Here's how the part is built. I have some questions about the finished solid (model axes, mm). A direction names the side the tool comes from. Round coordinates to 2 decimals unless told otherwise and drop trailing zeros. Order: outer loops, then holes, each group sorted by start corner. A loop starts at its lowest first (then second) coordinate and runs counter-clockwise, first axis right, second up. Notation, with made-up numbers: (14, 64) -> (30, 64) arc R36 ccw to (30, 98) -> close; hole circle Ø5 at (36, -27). An arc over 180 degrees is marked (long way). Use a Markdown table: item, result. Add a question column.
from build123d import *

# Parameters (mm, degrees)
BOSS_EXTRUDE1_DEPTH = 40
FILLET1_R           = 1
BOSS_EXTRUDE2_DEPTH = 7.5


with BuildPart() as part:
    # Sketch1 → Boss-Extrude1 (new body)
    with BuildSketch(Plane(origin=(0, 0, 0), x_dir=(1, 0, 0), z_dir=(0, 1, 0))):
        Polygon((0, 17.282938314), (-16.6777552, -7.65403186), (13.257172065, -9.628906454), align=None)
        Polygon((-0.263316613, 13.291614679), (-13.089509231, -5.886408918), (9.932242708, -7.405205761), align=None, mode=Mode.SUBTRACT)
    extrude(amount=BOSS_EXTRUDE1_DEPTH)

    # Fillet1
    fillet1_edges = [part.edges().sort_by_distance(p)[0] for p in [
        (9.932242708, 20, 7.405205761),
        (-0.263316613, 20, -13.291614679),
        (-13.089509231, 20, 5.886408918),
        (13.257172065, 20, 9.628906454),
        (-16.6777552, 20, 7.65403186),
        (0, 20, -17.282938314),
    ]]
    fillet(fillet1_edges, radius=FILLET1_R)

    # Sketch2 → Boss-Extrude2 (add, symmetric)
    with BuildSketch(Plane(origin=(0, 20, 0), x_dir=(-1, 0, 0), z_dir=(0, -1, 0))):
        Polygon((18.471878185, -8.537843331), (-14.919636743, -10.740756801), (-0.131658306, 19.278600132), align=None)
        with BuildLine():
            Line((-12.491768879, -8.075150372), (-0.765403186, 15.729182232))
            ThreePointArc((-0.765403186, 15.729182232), (0.065829153, 16.285107406), (0.962890645, 15.84320167))
            Line((0.962890645, 15.84320167), (15.714864555, -6.214295216))
            ThreePointArc((15.714864555, -6.214295216), (15.780693708, -7.212126125), (14.949461369, -7.768051298))
            Line((14.949461369, -7.768051298), (-11.528878233, -9.514887016))
            ThreePointArc((-11.528878233, -9.514887016), (-12.425939725, -9.072981281), (-12.491768879, -8.075150372))
        make_face(mode=Mode.SUBTRACT)
    extrude(amount=BOSS_EXTRUDE2_DEPTH, both=True)


solid = part.part
(1) I'm going to push flat-ended pins straight in: P1, Ø5, axis at y = 22, z = 1, coming from the -X side; P2, Ø10, axis at x = -9.5, y = 4.5, coming from the -Z side; P3, Ø12, axis at y = 23, z = -3.5, coming from the -X side. Where does each tip first touch, or does it pass through?
(2) I want a section at B-B on x = -8. List the corners of the cut face in (y, z) for me.
(3) If we mould it in two halves opening along Z, with no side actions, what happens to faces 5 (the flat face through (-1.9, 6.16, 8.63)), 6 (the cylindrical face through (-15.787, 33.838, 7.199)), 7 (the cylindrical face through (-12.2, 20.28, 5.43)), 8 (the flat face through (7.63, 19.9, -4.06))? For each: pulls with the +Z half, pulls with the -Z half, needs draft (parallel to the pull), parting line crosses it, or undercut.
(4) I want a section at D-D on x = -13. List the corners of the cut face in (y, z) for me, and give its area (3 significant figures).
(5) Please list where these lines run through material, in increasing order: probe 1 along Y at (x, z) = (-16, 7.5); probe 2 along Z at (x, y) = (6, 38.5); probe 3 along Z at (x, y) = (-11.5, 6). Write a range as from..to.
(6) I want a section at C-C on z = -2.5. List the corners of the cut face in (x, y) for me.
(7) I want a section at A-A on y = 12. List the corners of the cut face in (x, z) for me.
(8) On a 3-axis mill with a long thin cutter (end or side, diameter ignored), from which of +Z, -Z, +X, -X, +Y, -Y can I reach the whole of each face in a straight line? I mean faces 1 (the flat face through (6.71, 33.66, -3.66)), 2 (the cylindrical face through (-0.08, 6.338, -16.286)), 3 (the flat face through (-8.236, 33.662, -4.969)), 4 (the flat face through (7, 12.5, -4)). Say none if no direction works.
Output:
| question | item | result |
|---|---|---|
| 1 | P1 | x = -15.1 |
| 1 | P2 | z = -10.55 |
| 1 | P3 | x = -14.43 |
| 2 | outline | (0, -5.32) -> (12.5, -5.32) -> (12.5, -7.12) -> (27.5, -7.12) -> (27.5, -5.32) -> (40, -5.32) -> (40, -1.72) -> (0, -1.72) -> close; (0, 6.22) -> (40, 6.22) -> (40, 8.23) -> (27.5, 8.23) -> (27.5, 9.23) -> (12.5, 9.23) -> (12.5, 8.23) -> (0, 8.23) -> close |
| 3 | face 5 | pulls with the +Z half |
| 3 | face 6 | parting line crosses it |
| 3 | face 7 | undercut |
| 3 | face 8 | pulls with the -Z half |
| 4 | outline | (0, 2.15) -> (12.5, 2.15) -> (12.5, 0.36) -> (27.5, 0.36) -> (27.5, 2.15) -> (40, 2.15) -> (40, 7.9) -> (27.5, 7.9) -> (27.5, 8.9) -> (12.5, 8.9) -> (12.5, 7.9) -> (0, 7.9) -> close |
| 4 | area | 272 mm² |
| 5 | probe 1 | 12.5..27.5 |
| 5 | probe 2 | -5.1..-0.58, 7.15..9.15 |
| 5 | probe 3 | -0.09..3.51, 5.98..8 |
| 6 | outline | (-11.09, 12.5) -> (-9.89, 12.5) -> (-9.89, 0) -> (-7.48, 0) -> (-7.48, 40) -> (-9.89, 40) -> (-9.89, 27.5) -> (-11.09, 27.5) -> close; (5.05, 0) -> (7.28, 0) -> (7.28, 12.5) -> (8.4, 12.5) -> (8.4, 27.5) -> (7.28, 27.5) -> (7.28, 40) -> (5.05, 40) -> close |
| 7 | outline | (-15.71, 6.21) -> (-0.96, -15.84) arc R1 ccw to (0.77, -15.73) -> (12.49, 8.08) arc R1 ccw to (11.53, 9.51) -> (-14.95, 7.77) arc R1 ccw to start; hole (-12.13, 4.45) -> (-1.23, -11.85) arc R1 ccw to (0.5, -11.74) -> (9.17, 5.85) arc R1 ccw to (8.2, 7.29) -> (-11.36, 6) arc R1 ccw to start |
| 8 | face 1 | -Z, +X, +Y |
| 8 | face 2 | -Z, -Y |
| 8 | face 3 | -Z, -X, +Y |
| 8 | face 4 | -Y |
